Could you check a few things on this model? Use its own coordinates, in mm. Face numbers are marked on the shaded views. A direction names the side the tool comes from. Round coordinates to 2 decimals unless told otherwise and drop trailing zeros. Loops run counter-clockwise (first coordinate to the right, second up) from the corner with the lowest first, then second, coordinate; pieces in that order, holes last. Notation, with made-up numbers: (52, 48.25) -> (73, 48.25) arc R21 cw to (73, 68.25) -> close; hole circle Ø1 at (41, 46.5). An arc over 180 degrees is marked (long way). Use CSV: the item, a comma, the result in double quotes. Start each with the question number.
```python
from build123d import *

# Parameters (mm, degrees)
SKETCH1_R           = 4
BOSS_EXTRUDE1_DEPTH = 5.5
SKETCH2_R           = 6.5
SKETCH2_R_2         = 4
BOSS_EXTRUDE2_DEPTH = 2
FILLET1_R           = 2


with BuildPart() as part:
    # Sketch1 → Boss-Extrude1 (new body)
    with BuildSketch(Plane(origin=(0, 0, 0), x_dir=(1, 0, 0), z_dir=(0, 1, 0))):
        Polygon((6.5, -3.75277675), (6.5, 3.75277675), (0, 7.505553499), (-6.5, 3.75277675), (-6.5, -3.75277675), (0, -7.505553499), align=None)
        with Locations(Location((0, 0, 0), (0, 0, 270))):
            Circle(SKETCH1_R, mode=Mode.SUBTRACT)
    extrude(amount=BOSS_EXTRUDE1_DEPTH)

    # Sketch2 → Boss-Extrude2 (add)
    with BuildSketch(Plane(origin=(0, 5.5, 0), x_dir=(1, 0, 0), z_dir=(0, 1, 0))):
        with Locations(Location((0, 0, 0), (0, 0, 60))):
            Circle(SKETCH2_R)
        with Locations(Location((0, 0, 0), (0, 0, 270))):
            Circle(SKETCH2_R_2, mode=Mode.SUBTRACT)
    extrude(amount=BOSS_EXTRUDE2_DEPTH)

    # Fillet1
    fillet1_edges = [part.edges().sort_by_distance(p)[0] for p in [
        (-3.25, 7.5, 5.629165125),
    ]]
    fillet(fillet1_edges, radius=FILLET1_R - 0.0001)  # a hair under: the kernel refuses the full size


solid = part.part
```
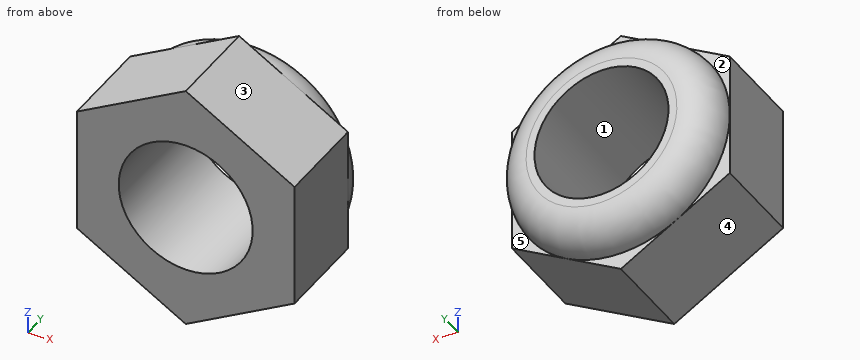
1. We'd pull the mould along X, two halves only. Please class the marked faces 1, 2 and 3: pulls with the +X half, pulls with the -X half, needs draft (parallel to the pull), parting line crosses it, or undercut.
2. Suppose I cut it at A-A (y = 2.75). List the corners of the cut face in (x, z) for me, then the cut area to 3 significant figures.
3. Suppose I cut it at C-C (y = 6.75). List the corners of the cut face in (x, z) for me, then the cut area to 3 significant figures.
4. Will these pins go through, and if not, where does the flat tip stop? pin 1 (0.9 mm diameter, centred on x = 0, z = -7, fed in from +Y); pin 2 (2 mm diameter, centred on x = -0.5, z = 6.5, fed in from +Y); pin 3 (1 mm diameter, centred on y = 2, z = -4.5, fed in from -X).
5. If I drill on L1, parallel to X at y = 5, z = 0; L2, parallel to Z at x = -3, y = 3.75; L3, parallel to Z at x = 2, y = 6.75, over which ranges is the centre line in solid material (lowest first)?
6. For the marked faces 4 and 5, which set-ups out of +Z, -Z, +X, -X, +Y, -Y let a thin tool reach every point of the face, with its end or its side?
7. Suppose I cut it at B-B (y = 6). List the corners of the cut face in (x, z) for me, then the cut area to 3 significant figures.
Geometry check:
1,face 1,"undercut"
1,face 2,"needs draft"
1,face 3,"pulls with the +X half"
2,outline,"(-6.5, -3.75) -> (0, -7.51) -> (6.5, -3.75) -> (6.5, 3.75) -> (0, 7.51) -> (-6.5, 3.75) -> close; hole circle Ø8 at (0, 0)"
2,area,"96.1 mm²"
3,outline,"circle Ø12.12 at (0, 0); hole circle Ø8 at (0, 0)"
3,area,"65.2 mm²"
4,pin 1,"stops at y = 5.5"
4,pin 2,"stops at y = 7.22"
4,pin 3,"stops at x = -6.07"
5,L1,"x = -6.5 to -4, 4 to 6.5"
5,L2,"z = -5.77 to -2.65, 2.65 to 5.77"
5,L3,"z = -5.72 to -3.46, 3.46 to 5.72"
6,face 4,"-Z, -X, +Y, -Y"
6,face 5,"-Z, +X, +Y"
7,outline,"circle Ø12.87 at (0, 0); hole circle Ø8 at (0, 0)"
7,area,"79.9 mm²"
